```python
from build123d import *

# Parameters (mm, degrees)
CROQUIS1_R              = 14
CROQUIS1_R_2            = 4.05
SALIENTE_EXTRUIR1_DEPTH = 18.9
CHAFL_N1_SIZE           = 1
CORTAR_EXTRUIR1_REACH   = 44.671
REDONDEO1_R             = 2
MATRIZC1_COUNT          = 3
REDONDEO1_OF_MATRIZC1_R = 2
CROQUIS3_R              = 4
CORTAR_EXTRUIR2_DEPTH   = 29
SALIENTE_EXTRUIR2_START = -3
CROQUIS6_R              = 18
CROQUIS6_R_2            = 4.05
SALIENTE_EXTRUIR2_DEPTH = 3
CHAFL_N2_SIZE           = 0.5
REDONDEO2_R             = 1
CROQUIS12_R             = 5.55
CORTAR_EXTRUIR4_DEPTH   = 3


with BuildPart() as part:
    # Croquis1 → Saliente-Extruir1 (new, symmetric)
    with BuildSketch(Plane(origin=(0, 0, 0), x_dir=(0, 1, 0), z_dir=(0, 0, 1))):
        with Locations(Location((0, 0, 0), (0, 0, 270))):
            Circle(CROQUIS1_R)
        with Locations(Location((0, 0, 0), (0, 0, 270))):
            Circle(CROQUIS1_R_2, mode=Mode.SUBTRACT)
    extrude(amount=SALIENTE_EXTRUIR1_DEPTH, both=True)

    # Chaflán1
    chafl_n1_edges = [part.edges().sort_by_distance(p)[0] for p in [
        (-14, 0, 18.9),
    ]]
    chamfer(chafl_n1_edges, length=CHAFL_N1_SIZE)

    # Croquis2 → Cortar-Extruir1 (cut, up to next)
    with BuildSketch(Plane.XY.offset(18.9), mode=Mode.PRIVATE) as cortar_extruir1_sk1:
        with BuildLine():
            Line((4.729506573, 4.458897574), (4.781865786, 10.458669113))
            ThreePointArc((4.781865786, 10.458669113), (0, 11.5), (-4.781865786, 10.458669113))
            Line((-4.781865786, 10.458669113), (-4.729506573, 4.458897574))
            ThreePointArc((-4.729506573, 4.458897574), (0, 6.5), (4.729506573, 4.458897574))
        make_face()
    cortar_extruir1_tool1 = extrude(cortar_extruir1_sk1.sketch, amount=-CORTAR_EXTRUIR1_REACH, mode=Mode.PRIVATE) & part.part
    cortar_extruir1 = cortar_extruir1_tool1.solids().sort_by_distance((0, 8.49359, 18.9))[0]
    add(cortar_extruir1, mode=Mode.SUBTRACT)

    # Redondeo1
    redondeo1_edges = [part.edges().sort_by_distance(p)[0] for p in [
        (4.729506573, 4.458897574, 0),
        (-4.729506573, 4.458897574, 0),
        (-4.781865786, 10.458669113, 0),
        (4.781865786, 10.458669113, 0),
    ]]
    fillet(redondeo1_edges, radius=REDONDEO1_R)

    # MatrizC1: Cortar-Extruir1 ×3 about axis
    matrizc1_axis = Axis((0, 0, 0), (0, 0, 1))
    for i in range(1, MATRIZC1_COUNT):
        add(cortar_extruir1.rotate(matrizc1_axis, i * 360 / MATRIZC1_COUNT), mode=Mode.SUBTRACT)

    # Redondeo1 of MatrizC1
    redondeo1_of_matrizc1_edges = [part.edges().sort_by_distance(p)[0] for p in [
        (-6.226271859, 1.866424052, 0),
        (-1.496765286, -6.325321627, 0),
        (-6.666540248, -9.370551804, 0),
        (-11.448406034, -1.088117308, 0),
        (1.496765286, -6.325321627, 0),
        (6.226271859, 1.866424052, 0),
        (11.448406034, -1.088117308, 0),
        (6.666540248, -9.370551804, 0),
    ]]
    fillet(redondeo1_of_matrizc1_edges, radius=REDONDEO1_OF_MATRIZC1_R)

    # Croquis3 → Cortar-Extruir2 (cut)
    with BuildSketch(Plane(origin=(0, 0, 0), x_dir=(-1, 0, 0), z_dir=(0, 1, 0))):
        with Locations(Location((0, -0.4, 0), (0, 0, 90))):
            Circle(CROQUIS3_R)
    extrude(amount=-CORTAR_EXTRUIR2_DEPTH, mode=Mode.SUBTRACT)

    # Croquis6 → Saliente-Extruir2 (add)
    with BuildSketch(Plane(origin=(0, 0, -18.9), x_dir=(1, 0, 0), z_dir=(0, 0, -1)).offset(SALIENTE_EXTRUIR2_START)):
        with Locations(Location((0, 0, 0), (0, 0, 180))):
            Circle(CROQUIS6_R)
        Circle(CROQUIS6_R_2, mode=Mode.SUBTRACT)
        with BuildLine():
            Line((-10.239546073, 0.40417725), (-9.32733269, -0.111928251))
            ThreePointArc((-9.32733269, -0.111928251), (-7.50591795, -0.187849628), (-6.379547789, 1.245540049))
            ThreePointArc((-6.379547789, 1.245540049), (-5.629165125, 3.25), (-4.268443218, 4.902080425))
            ThreePointArc((-4.268443218, 4.902080425), (-3.590276425, 6.594240438), (-4.566733636, 8.133671184))
            Line((-4.566733636, 8.133671184), (-5.469800803, 8.665618398))
            ThreePointArc((-5.469800803, 8.665618398), (-6.703454741, 8.930380198), (-7.850114903, 8.403909567))
            ThreePointArc((-7.850114903, 8.403909567), (-9.959292144, 5.75), (-11.203056628, 2.596444145))
            ThreePointArc((-11.203056628, 2.596444145), (-11.085663488, 1.340172), (-10.239546073, 0.40417725))
        make_face(mode=Mode.SUBTRACT)
        with BuildLine():
            Line((5.469800803, 8.665618398), (4.566733636, 8.133671184))
            ThreePointArc((4.566733636, 8.133671184), (3.590276425, 6.594240438), (4.268443218, 4.902080425))
            ThreePointArc((4.268443218, 4.902080425), (5.629165125, 3.25), (6.379547789, 1.245540049))
            ThreePointArc((6.379547789, 1.245540049), (7.50591795, -0.187849628), (9.32733269, -0.111928251))
            Line((9.32733269, -0.111928251), (10.239546073, 0.40417725))
            ThreePointArc((10.239546073, 0.40417725), (11.085663488, 1.340172), (11.203056628, 2.596444145))
            ThreePointArc((11.203056628, 2.596444145), (9.959292144, 5.75), (7.850114903, 8.403909567))
            ThreePointArc((7.850114903, 8.403909567), (6.703454741, 8.930380198), (5.469800803, 8.665618398))
        make_face(mode=Mode.SUBTRACT)
        with BuildLine():
            Line((-4.760599053, -8.021742934), (-4.769745271, -9.069795648))
            ThreePointArc((-4.769745271, -9.069795648), (-4.382208746, -10.270552198), (-3.352941725, -11.000353712))
            ThreePointArc((-3.352941725, -11.000353712), (0, -11.5), (3.352941725, -11.000353712))
            ThreePointArc((3.352941725, -11.000353712), (4.382208746, -10.270552198), (4.769745271, -9.069795648))
            Line((4.769745271, -9.069795648), (4.760599053, -8.021742934))
            ThreePointArc((4.760599053, -8.021742934), (3.915641525, -6.40639081), (2.11110457, -6.147620474))
            ThreePointArc((2.11110457, -6.147620474), (0, -6.5), (-2.11110457, -6.147620474))
            ThreePointArc((-2.11110457, -6.147620474), (-3.915641525, -6.40639081), (-4.760599053, -8.021742934))
        make_face(mode=Mode.SUBTRACT)
    extrude(amount=SALIENTE_EXTRUIR2_DEPTH)

    # Chaflán2
    chafl_n2_edges = [part.edges().sort_by_distance(p)[0] for p in [
        (18, 0, -18.9),
        (18, 0, -15.9),
    ]]
    chamfer(chafl_n2_edges, length=CHAFL_N2_SIZE)

    # Redondeo2
    redondeo2_edges = [part.edges().sort_by_distance(p)[0] for p in [
        (-14, 0, -15.9),
    ]]
    fillet(redondeo2_edges, radius=REDONDEO2_R)

    # Croquis12 → Cortar-Extruir4 (cut)
    with BuildSketch(Plane.XY.offset(18.9)):
        Circle(CROQUIS12_R)
    extrude(amount=-CORTAR_EXTRUIR4_DEPTH, mode=Mode.SUBTRACT)


solid = part.part
```
Work out the finished part from the listing and answer in its coordinate system (mm). A direction names the side the tool comes from. Give positions to 0.01 mm unless a question says otherwise; leave off trailing zeros. Order: outer loops, then holes, each group sorted by start corner. A loop starts at its lowest first (then second) coordinate and runs counter-clockwise, first axis right, second up. Notation, with made-up numbers: (7, 76) -> (66, 76) arc R12 ccw to (66, 89) -> close; hole circle Ø5 at (-37, 72). An arc over 180 degrees is marked (long way). Answer as CSV lines item,"result". Start each with the question number.
(1) Section B-B, the plane z = 14.5 is taken. Write down the section's boundary in (x, y), plus the area to 3 significant figures.
(2) Consider line 1 along X through (y, z) = (-0.5, -3.5); line 2 along X through (y, z) = (-3, 11.5); line 3 along X through (y, z) = (1, -12). Determine where each line is inside the solid, lowest interval first.
(3) For a pull along X with two mould halves and no side action, classify faces 1 (the flat face through (-13, 8, -15.9)), 2 (the cylindrical face through (-3.937, 6.422, -0.265)) as released by +X, released by -X, zero draft, split by the parting line, or undercut.
(4) Which of the six approach directions +Z, -Z, +X, -X, +Y, -Y give full straight-line access (tool end or side, diameter ignored) to faces 3 (the cylindrical face through (-1.532, -8.702, 3.295)), 4 (the flat face through (-4, -4, -18.9)), 5 (the cylindrical face through (-4.41, -8.03, -0.26))?
(5) Section A-A, the plane x = 0 is taken. Give the number of separate pieces and of enclosed holes in the cut face, plus the area to 3 significant figures.
(6) Each of these flat-tipped pins is pushed along its axis until it touches: pin 1 Ø12 at (y, z) = (-0.5, -10) entering from -X; pin 2 Ø7 at (x, z) = (0, -0.4) entering from +Y; pin 3 Ø12 at (x, y) = (-1.5, -2) entering from +Z; pin 4 Ø10 at (y, z) = (4, -2.5) entering from -X. Where does it stop, or does it pass through?
Entries:
1,outline,"circle Ø28 at (0, 0); hole (-11.2, -2.6) arc R11.5 ccw to (-7.85, -8.4) arc R2 ccw to (-5.47, -8.67) -> (-4.57, -8.13) arc R2 ccw to (-4.27, -4.9) arc R6.5 cw to (-6.38, -1.25) arc R2 ccw to (-9.33, 0.11) -> (-10.24, -0.4) arc R2 ccw to start; hole (-4.77, 9.07) -> (-4.76, 8.02) arc R2 ccw to (-2.11, 6.15) arc R6.5 cw to (2.11, 6.15) arc R2 ccw to (4.76, 8.02) -> (4.77, 9.07) arc R2 ccw to (3.35, 11) arc R11.5 ccw to (-3.35, 11) arc R2 ccw to start; hole circle Ø8.1 at (0, 0); hole (4.27, -4.9) arc R2 ccw to (4.57, -8.13) -> (5.47, -8.67) arc R2 ccw to (7.85, -8.4) arc R11.5 ccw to (11.2, -2.6) arc R2 ccw to (10.24, -0.4) -> (9.33, 0.11) arc R2 ccw to (6.38, -1.25) arc R6.5 cw to start"
1,area,"430 mm²"
2,line 1,"-13.99 to -10.39, -6.69 to -4.02, 4.02 to 6.69, 10.39 to 13.99"
2,line 2,"-13.67 to -11.1, -5.77 to -2.72, 2.72 to 5.77, 11.1 to 13.67"
2,line 3,"-13.96 to -3.92, 3.92 to 13.96"
3,face 1,"zero draft"
3,face 2,"undercut"
4,face 3,"-Y"
4,face 4,"-Z, +X, -X, +Y, -Y"
4,face 5,"+Z, -Z"
5,separate pieces,"4"
5,enclosed holes,"0"
5,area,"498 mm²"
6,pin 1,"x = -17.59"
6,pin 2,"y = 14"
6,pin 3,"z = 18.9"
6,pin 4,"x = -14"
